Autodesk Fusion 360 part; units mm, degrees
sketch "Skizze1" plane through (0, 0, 0) normal (0, 0, 1) x (1, 0, 0)
  circle A0 centre (0, 0) radius 35
  circle A1 centre (0, 0) radius 40
  line L0 (10, 30) -> (-10, 30)
  line L1 (-10, 30) -> (-10, 45)
  line L2 (-10, 45) -> (10, 45)
  line L3 (10, 45) -> (10, 30)
  line L4 (15, 35) -> (10, 35)
  line L5 (10, 35) -> (10, 45)
  line L6 (10, 45) -> (15, 45)
  line L7 (15, 45) -> (15, 35)
  line L8 (-10, 35) -> (-15, 35)
  line L9 (-15, 35) -> (-15, 45)
  line L10 (-15, 45) -> (-10, 45)
  line L11 (-10, 45) -> (-10, 35)
  line L12 (-15, -35) -> (15, -35)
  line L13 (15, -35) -> (15, -40)
  line L14 (15, -40) -> (-15, -40)
  line L15 (-15, -40) -> (-15, -35)
  dimension "d1" = 70
  dimension "d2" = 80
extrude "Extrusion1" add sketch "Skizze1" along normal blind 25 contours A0 A1 L3 L4 L7 L12 L13 | A0 A1 L1 L8 L9 L12 L15 | A1 L12 L13 L15 | A1 L3 L4 L5 L7 | A1 L1 L8 L9 L11 | A1 L3 L5 L6 L7 | A1 L14 L15 | A1 L13 L14 | A1 L1 L9 L10 L11
hole "Bohrung1" at (0, -40, 12.5) direction (0, 1, 0) diameter 13 depth 5 tip angle 118
Source: CAD feature listing. Evaluate the final solid. Frame: model axes, mm. A direction names the side the tool comes from. Round coordinates to 2 decimals unless told otherwise and drop trailing zeros. Write each loop counter-clockwise with the first axis right and the second up, starting at its lowest first coordinate (ties: lowest second). Pieces come first, ordered by that corner, then holes. Notation, with made-up numbers: (25.25, 23.5) - (32.25, 23.5) arc R23 ccw to (32.25, 49.5) - close; hole circle Ø5 at (32, -16). An arc over 180 degrees is marked (long way). Use CSV: the item, a comma, the result in double quotes. Start each with the question number.
(1) Set-up query: faces 5 (the face through (15, -39, 12)), 6 (the face through (-15, -39, 12)), 7 (the face through (-10, 39, 12)). Return all of +Z, -Z, +X, -X, +Y, -Y with unobstructed straight access to the full face (end or side cutting, diameter ignored); none if empty.
(2) First-contact query: pin 1 Ø2.5 at (y, z) = (41.5, 14.5) entering from -X; pin 2 Ø8 at (y, z) = (9, 21) entering from +X; pin 3 Ø3.5 at (y, z) = (42, 11) entering from +X; pin 4 Ø15 at (x, z) = (0, 12.5) entering from -Y. Flat tips, straight axial feed; report the tip coordinate or a pass-through.
(3) Cut plane D-D, the plane z = 12.5. Return loops of the section in (x, y), and give its area (3 significant figures).
(4) Mould query, pull axis Z, two halves, no side actions, for faces 1 (the face through (-1.95, -37.47, 6.3)), 2 (the face through (15, 41, 12)), 3 (the face through (5.939, -34.664, 12.369)), 4 (the face through (-3.1, -35.1, 25)). Classes: pulls with the +Z half, pulls with the -Z half, needs draft (parallel to the pull), parting line crosses it, or undercut.
(5) Cut plane B-B, the plane x = 25.5. Return loops of the section in (y, z).
(6) Cut plane C-C, the plane z = 23.25. Return loops of the section in (x, y), and give its area (3 significant figures).
(7) Cut plane A-A, the plane y = 0. Return loops of the section in (x, z).
(8) Material intervals for probe 1 along X at (y, z) = (-38.9, 12.5); probe 2 along Z at (x, y) = (0, -38.3); probe 3 along X at (y, z) = (0, 18.5), sorted ascending. Write a range as [from, to].
Geometry says:
1,face 5,"+Z, -Z, +X, -Y"
1,face 6,"+Z, -Z, -X, -Y"
1,face 7,"+Z, -Z, +Y"
2,pin 1,"x = -15"
2,pin 2,"x = 39.69"
2,pin 3,"x = 15"
2,pin 4,"y = -40"
3,outline,"(-15, -40) - (-6.5, -40) - (-6.5, -35) - (-5.72, -34.53) arc R35 cw to (-10, 33.54) - (-10, 45) - (-15, 45) - (-15, 37.08) arc R40 ccw to (-15, -37.08) - close; (5.72, -34.53) - (6.5, -35) - (6.5, -40) - (15, -40) - (15, -37.08) arc R40 ccw to (15, 37.08) - (15, 45) - (10, 45) - (10, 33.54) arc R35 cw to start"
3,area,"1,110 mm²"
4,face 1,"undercut"
4,face 2,"needs draft"
4,face 3,"undercut"
4,face 4,"pulls with the +Z half"
5,outline,"(-30.82, 0) - (-23.97, 0) - (-23.97, 25) - (-30.82, 25) - close; (23.97, 0) - (30.82, 0) - (30.82, 25) - (23.97, 25) - close"
6,outline,"(-15, -40) - (15, -40) - (15, -37.08) arc R40 ccw to (15, 37.08) - (15, 45) - (10, 45) - (10, 33.54) arc R35 cw (long way) to (-10, 33.54) - (-10, 45) - (-15, 45) - (-15, 37.08) arc R40 ccw to (-15, -37.08) - close"
6,area,"1,180 mm²"
7,outline,"(-40, 0) - (-35, 0) - (-35, 25) - (-40, 25) - close; (35, 0) - (40, 0) - (40, 25) - (35, 25) - close"
8,probe 1,"[-15, -6.5], [6.5, 15]"
8,probe 2,"[0, 6], [19, 25]"
8,probe 3,"[-40, -35], [35, 40]"
